Part print with two shaded views. Sizes in mm from the minimum x, y, z corner. Coordinates: 2 decimals unless noted, no trailing zeros. Write each loop counter-clockwise with the first axis right and the second up, starting at its lowest first coordinate (ties: lowest second). Pieces come first, ordered by that corner, then holes. Notation, with made-up numbers: (-6, 77) - (9, 77) arc R21 ccw to (9, 96) - close; hole circle Ø2 at (-32, 41.5). An arc over 180 degrees is marked (long way). Answer in a Markdown table with one row per item. Add a question column.
Q1. Two-plate mould, pull along X, no slides. Class the marked faces 1, 2, 3 and 4: +X half, -X half, draft (parallel to the pull), parting line (faces both ways), or undercut.
Q2. Band-saw the part on B-B (x = 18). List the corners of the cut face in (y, z) (1 decimal).
Q3. Pin check, flat tip, straight feed: pin 1 (8.5 mm diameter, centred on y = 10.16, z = 10.16, fed in from +X). Stop position of the tip, or through.
Q4. Drill centre lines: line 1 along Y through (x, z) = (17.25, 10.25); line 2 along Y through (x, z) = (19, 7.5). Where is each one in solid material? Low to high. Write a range as from..to.
Q5. Band-saw the part on A-A (y = 10.16). List the corners of the cut face in (x, z), and give its area (3 significant figures).
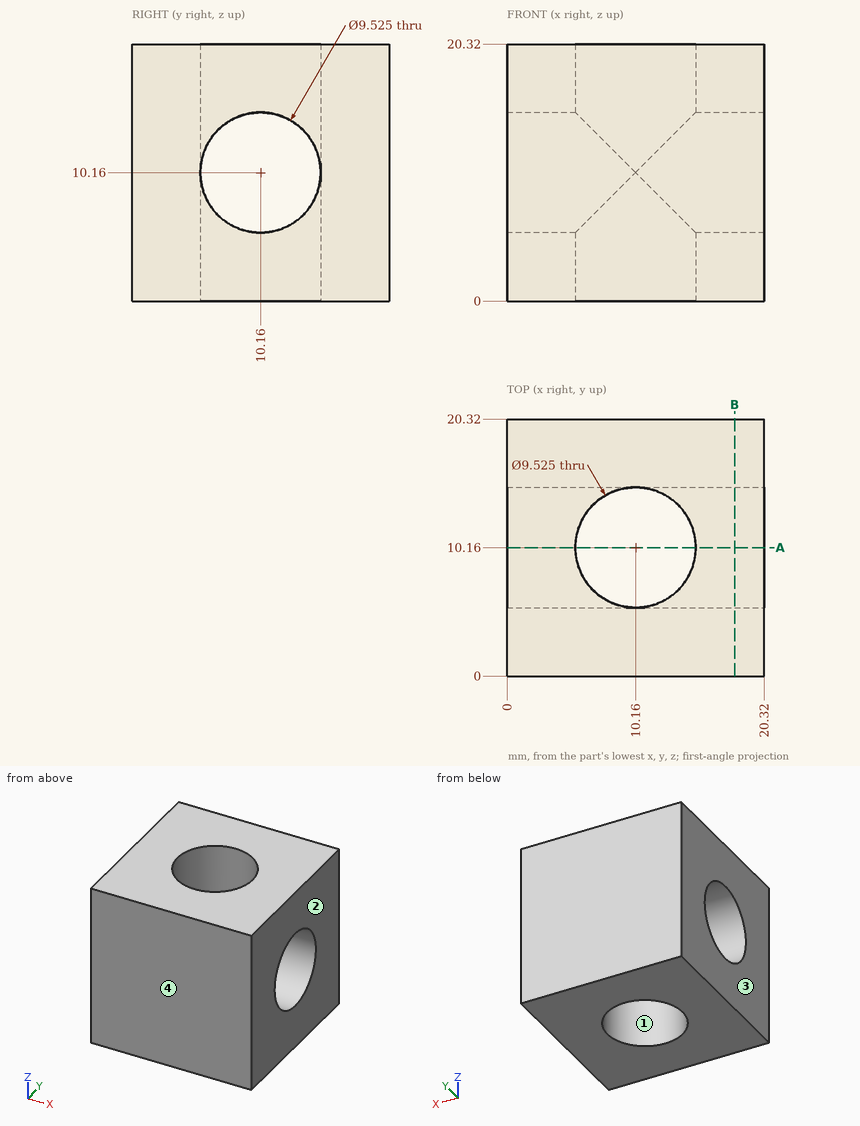
Checked values:
| question | item | result |
|---|---|---|
| 1 | face 1 | undercut |
| 1 | face 2 | +X half |
| 1 | face 3 | -X half |
| 1 | face 4 | draft |
| 2 | outline | (0, 0) - (20.3, 0) - (20.3, 20.3) - (0, 20.3) - close; hole circle Ø9.5 at (10.2, 10.2) |
| 3 | pin 1 | passes through |
| 4 | line 1 | y = 0..5.4, 14.92..20.32 |
| 4 | line 2 | y = 0..6.21, 14.11..20.32 |
| 5 | outline | (0, 0) - (5.4, 0) - (5.4, 5.4) - (0, 5.4) - close; (0, 14.92) - (5.4, 14.92) - (5.4, 20.32) - (0, 20.32) - close; (14.92, 0) - (20.32, 0) - (20.32, 5.4) - (14.92, 5.4) - close; (14.92, 14.92) - (20.32, 14.92) - (20.32, 20.32) - (14.92, 20.32) - close |
| 5 | area | 117 mm² |
